from build123d import *

# Parameters (mm, degrees)
SKETCH1_W           = 150
SKETCH1_H           = 150
BOSS_EXTRUDE1_DEPTH = 300
SKETCH2_W           = 130
SKETCH2_H           = 135
CUT_EXTRUDE1_DEPTH  = 130
SKETCH3_W           = 10
SKETCH3_H           = 30
BOSS_EXTRUDE2_DEPTH = 10
SKETCH4_R           = 2.5
CUT_EXTRUDE2_DEPTH  = 344.365694268
FILLET1_RADIUS      = 5
FILLET1_LENGTH      = 30
FILLET2_RADIUS      = 5
FILLET2_LENGTH      = 30
FILLET3_RADIUS      = 5
FILLET3_LENGTH      = 30
FILLET4_RADIUS      = 5
FILLET4_LENGTH      = 30
FILLET5_RADIUS      = 5
FILLET5_LENGTH      = 30
SKETCH5_W           = 3.175
SKETCH5_H           = 20
BOSS_EXTRUDE3_DEPTH = 20


with BuildPart() as part:
    # Sketch1 → Boss-Extrude1 (new body)
    with BuildSketch(Plane(origin=(0, 0, 0), x_dir=(1, 0, 0), z_dir=(0, 1, 0))):
        with Locations((75, 75)):
            Rectangle(SKETCH1_W, SKETCH1_H)
    extrude(amount=BOSS_EXTRUDE1_DEPTH)

    # Sketch2 → Cut-Extrude1 (cut)
    with BuildSketch(Plane.XY):
        with Locations((75, 77.5)):
            Rectangle(SKETCH2_W, SKETCH2_H)
        with Locations((75, 222.5)):
            Rectangle(SKETCH2_W, SKETCH2_H)
    extrude(amount=-CUT_EXTRUDE1_DEPTH, mode=Mode.SUBTRACT)

    # Sketch3 → Boss-Extrude2 (add)
    with BuildSketch(Plane.ZY):
        with Locations((5, 75)):
            Rectangle(SKETCH3_W, SKETCH3_H)
        with Locations((5, 15)):
            Rectangle(SKETCH3_W, SKETCH3_H)
        with Locations((5, 135)):
            Rectangle(SKETCH3_W, SKETCH3_H)
        with Locations((5, 195)):
            Rectangle(SKETCH3_W, SKETCH3_H)
        with Locations((5, 255)):
            Rectangle(SKETCH3_W, SKETCH3_H)
    extrude(amount=-BOSS_EXTRUDE2_DEPTH)

    # Sketch4 → Cut-Extrude2 (cut, through all)
    with BuildSketch(Plane(origin=(0, 270, 0), x_dir=(1, 0, 0), z_dir=(0, 1, 0))):
        with Locations(Location((5, -5, 0), (0, 0, 270))):
            Circle(SKETCH4_R)
    extrude(amount=-CUT_EXTRUDE2_DEPTH, mode=Mode.SUBTRACT)

    # Fillet1: full round fillet: the end face becomes a half cylinder, R = half its width
    fillet1_face = Plane((5, 255, 10), x_dir=(0, 1, 0), z_dir=(0, 0, 1))  # on the end face: x along it, z out of the body
    fillet1_slab = fillet1_face.offset(-FILLET1_RADIUS / 2) * Box(FILLET1_LENGTH, 2 * FILLET1_RADIUS, FILLET1_RADIUS, mode=Mode.PRIVATE)  # the body's end, R deep
    fillet1_round = Plane((5, 255, 5), x_dir=(0, 0, 1), z_dir=(0, 1, 0)) * Cylinder(FILLET1_RADIUS, FILLET1_LENGTH, mode=Mode.PRIVATE)  # its axis R under the face
    add(fillet1_slab - fillet1_round, mode=Mode.SUBTRACT)

    # Fillet2: full round fillet: the end face becomes a half cylinder, R = half its width
    fillet2_face = Plane((5, 195, 10), x_dir=(0, 1, 0), z_dir=(0, 0, 1))  # on the end face: x along it, z out of the body
    fillet2_slab = fillet2_face.offset(-FILLET2_RADIUS / 2) * Box(FILLET2_LENGTH, 2 * FILLET2_RADIUS, FILLET2_RADIUS, mode=Mode.PRIVATE)  # the body's end, R deep
    fillet2_round = Plane((5, 195, 5), x_dir=(0, 0, 1), z_dir=(0, 1, 0)) * Cylinder(FILLET2_RADIUS, FILLET2_LENGTH, mode=Mode.PRIVATE)  # its axis R under the face
    add(fillet2_slab - fillet2_round, mode=Mode.SUBTRACT)

    # Fillet3: full round fillet: the end face becomes a half cylinder, R = half its width
    fillet3_face = Plane((5, 135, 10), x_dir=(0, 1, 0), z_dir=(0, 0, 1))  # on the end face: x along it, z out of the body
    fillet3_slab = fillet3_face.offset(-FILLET3_RADIUS / 2) * Box(FILLET3_LENGTH, 2 * FILLET3_RADIUS, FILLET3_RADIUS, mode=Mode.PRIVATE)  # the body's end, R deep
    fillet3_round = Plane((5, 135, 5), x_dir=(0, 0, 1), z_dir=(0, 1, 0)) * Cylinder(FILLET3_RADIUS, FILLET3_LENGTH, mode=Mode.PRIVATE)  # its axis R under the face
    add(fillet3_slab - fillet3_round, mode=Mode.SUBTRACT)

    # Fillet4: full round fillet: the end face becomes a half cylinder, R = half its width
    fillet4_face = Plane((5, 75, 10), x_dir=(0, 1, 0), z_dir=(0, 0, 1))  # on the end face: x along it, z out of the body
    fillet4_slab = fillet4_face.offset(-FILLET4_RADIUS / 2) * Box(FILLET4_LENGTH, 2 * FILLET4_RADIUS, FILLET4_RADIUS, mode=Mode.PRIVATE)  # the body's end, R deep
    fillet4_round = Plane((5, 75, 5), x_dir=(0, 0, 1), z_dir=(0, 1, 0)) * Cylinder(FILLET4_RADIUS, FILLET4_LENGTH, mode=Mode.PRIVATE)  # its axis R under the face
    add(fillet4_slab - fillet4_round, mode=Mode.SUBTRACT)

    # Fillet5: full round fillet: the end face becomes a half cylinder, R = half its width
    fillet5_face = Plane((5, 15, 10), x_dir=(0, 1, 0), z_dir=(0, 0, 1))  # on the end face: x along it, z out of the body
    fillet5_slab = fillet5_face.offset(-FILLET5_RADIUS / 2) * Box(FILLET5_LENGTH, 2 * FILLET5_RADIUS, FILLET5_RADIUS, mode=Mode.PRIVATE)  # the body's end, R deep
    fillet5_round = Plane((5, 15, 5), x_dir=(0, 0, 1), z_dir=(0, 1, 0)) * Cylinder(FILLET5_RADIUS, FILLET5_LENGTH, mode=Mode.PRIVATE)  # its axis R under the face
    add(fillet5_slab - fillet5_round, mode=Mode.SUBTRACT)

    # Sketch5 → Boss-Extrude3 (add)
    with BuildSketch(Plane.XZ):
        with Locations((1.5875, -140)):
            Rectangle(SKETCH5_W, SKETCH5_H)
        with Locations((1.5875, -10)):
            Rectangle(SKETCH5_W, SKETCH5_H)
        with Locations((148.4125, -10)):
            Rectangle(SKETCH5_W, SKETCH5_H)
        with Locations((148.4125, -140)):
            Rectangle(SKETCH5_W, SKETCH5_H)
    extrude(amount=BOSS_EXTRUDE3_DEPTH)


solid = part.part
Source: CAD feature listing. Evaluate the final solid. Frame: model axes, mm. A direction names the side the tool comes from. Round coordinates to 2 decimals unless told otherwise and drop trailing zeros. Loops run counter-clockwise (first coordinate to the right, second up) from the corner with the lowest first, then second, coordinate; pieces in that order, holes last.
Q1. Access query for faces 4 (the face through (74, 300, -76)), 5 (the face through (3, 60, 3)), 6 (the face through (10, 222, -62)), 7 (the face through (3.175, -10, -10)). Directions: +Z, -Z, +X, -X, +Y, -Y. A direction counts if a zero-diameter tool reaches every point of the face in a straight line with its end or side. Return the directions, or none.
Q2. Ray query, line 1 (Y direction, x = 84, z = -90.5); line 2 (X direction, y = 118, z = -67); line 3 (X direction, y = 144, z = 5). Return the intervals inside material, ascending.
Q3. Section A-A, the plane y = 14.5. Return loops of the section in (x, z).
Q4. Section D-D, the plane z = -11.5. Return loops of the section in (x, y) (3 decimals).
Q5. Mould query, pull axis X, two halves, no side actions, for faces 1 (the face through (146.825, -10, -10)), 2 (the face through (150, 138, -74)), 3 (the face through (3, 180, 3)). Classes: pulls with the +X half, pulls with the -X half, needs draft (parallel to the pull), parting line crosses it, or undercut.
Q6. First-contact query: P1, Ø1, axis at x = 132, z = -21, coming from the -Y side; P2, Ø11, axis at x = 5, y = 51, coming from the +Z side; P3, Ø11, axis at x = 7, z = 6, coming from the +Y side. Flat tips, straight axial feed; report the tip coordinate or a pass-through.
Q7. Section B-B, the plane z = -47. Return loops of the section in (x, y), plus the area to 3 significant figures.
Q8. Section C-C, the plane x = 22.5. Return loops of the section in (y, z).
Solutions:
1. face 4: +Z, -Z, +X, -X, +Y
1. face 5: +Z, +X, -X
1. face 6: +Z
1. face 7: +Z, -Z, -Y
2. line 1: y = 0 to 10, 145 to 155, 290 to 300
2. line 2: x = 0 to 10, 140 to 150
2. line 3: x = 0 to 2.5, 7.5 to 10
3. outline: (0, -150) - (150, -150) - (150, 0) - (140, 0) - (140, -130) - (10, -130) - (10, 5) arc R5 ccw to (0, 5) - close; hole circle Ø5 at (5, 5)
4. outline: (0, -20) - (3.175, -20) - (3.175, 0) - (146.825, 0) - (146.825, -20) - (150, -20) - (150, 300) - (0, 300) - close; hole (10, 10) - (140, 10) - (140, 145) - (10, 145) - close; hole (10, 155) - (140, 155) - (140, 290) - (10, 290) - close
5. face 1: undercut
5. face 2: pulls with the +X half
5. face 3: needs draft
6. P1: stops at y = 0
6. P2: stops at z = 0
6. P3: stops at y = 270
7. outline: (0, 0) - (150, 0) - (150, 300) - (0, 300) - close; hole (10, 10) - (140, 10) - (140, 145) - (10, 145) - close; hole (10, 155) - (140, 155) - (140, 290) - (10, 290) - close
7. area: 9,900 mm2
8. outline: (0, -150) - (300, -150) - (300, 0) - (290, 0) - (290, -130) - (155, -130) - (155, 0) - (145, 0) - (145, -130) - (10, -130) - (10, 0) - (0, 0) - close
